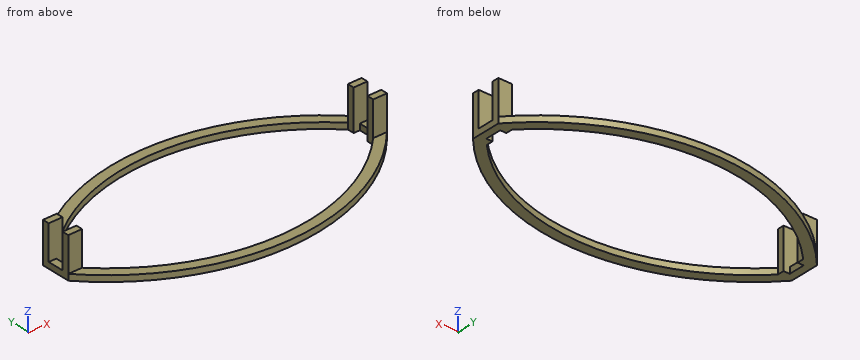
from build123d import *

# Parameters (mm, degrees)
F0_W     = 3.75
F0_H     = 8
F1_DEPTH = 3
F2_DEPTH = 20


with BuildPart() as f1:
    # F0 (on Top) → F1 (new body)
    with BuildSketch(Plane.XY):
        with BuildLine():
            Line((-3.75, 11.307189), (3.051668, 11.307189))
            ThreePointArc((3.051668, 11.307189), (75, 41.856217), (146.948332, 11.307189))
            Line((146.948332, 11.307189), (153.75, 11.307189))
            ThreePointArc((153.75, 11.307189), (75, 46.856217), (-3.75, 11.307189))
        make_face()
        with BuildLine():
            ThreePointArc((146.948332, -3.307189), (75, -33.856217), (3.051668, -3.307189))
            Line((3.051668, -3.307189), (-3.75, -3.307189))
            ThreePointArc((-3.75, -3.307189), (75, -38.856217), (153.75, -3.307189))
            Line((153.75, -3.307189), (146.948332, -3.307189))
        make_face()
        with Locations((151.875, 4)):
            Rectangle(F0_W, F0_H)
        with Locations((-1.875, 4)):
            Rectangle(F0_W, F0_H)
    extrude(amount=F1_DEPTH)

    # F0 (on Top) → F2 (join)
    with BuildSketch(Plane.XY):
        with BuildLine():
            Line((-3.75, 8), (0, 8))
            ThreePointArc((0, 8), (1.507229, 9.670762), (3.051668, 11.307189))
            Line((3.051668, 11.307189), (-3.75, 11.307189))
            Line((-3.75, 11.307189), (-3.75, 8))
        make_face()
        with BuildLine():
            ThreePointArc((3.051668, 11.307189), (1.507229, 9.670762), (0, 8))
            Line((0, 8), (3.051668, 8))
            Line((3.051668, 8), (3.051668, 11.307189))
        make_face()
        with BuildLine():
            ThreePointArc((3.051668, -3.307189), (1.507229, -1.670762), (0, 0))
            Line((0, 0), (-3.75, 0))
            Line((-3.75, 0), (-3.75, -3.307189))
            Line((-3.75, -3.307189), (3.051668, -3.307189))
        make_face()
        with BuildLine():
            Line((3.051668, 0), (0, 0))
            ThreePointArc((0, 0), (1.507229, -1.670762), (3.051668, -3.307189))
            Line((3.051668, -3.307189), (3.051668, 0))
        make_face()
        with BuildLine():
            Line((153.75, 11.307189), (146.948332, 11.307189))
            ThreePointArc((146.948332, 11.307189), (148.492771, 9.670762), (150, 8))
            Line((150, 8), (153.75, 8))
            Line((153.75, 8), (153.75, 11.307189))
        make_face()
        with BuildLine():
            ThreePointArc((150, 8), (148.492771, 9.670762), (146.948332, 11.307189))
            Line((146.948332, 11.307189), (146.948332, 8))
            Line((146.948332, 8), (150, 8))
        make_face()
        with BuildLine():
            ThreePointArc((150, 0), (148.492771, -1.670762), (146.948332, -3.307189))
            Line((146.948332, -3.307189), (153.75, -3.307189))
            Line((153.75, -3.307189), (153.75, 0))
            Line((153.75, 0), (150, 0))
        make_face()
        with BuildLine():
            Line((146.948332, 0), (146.948332, -3.307189))
            ThreePointArc((146.948332, -3.307189), (148.492771, -1.670762), (150, 0))
            Line((150, 0), (146.948332, 0))
        make_face()
    extrude(amount=F2_DEPTH)


solid = f1.part
The listing builds one solid part. Answer for the finished solid, in the listing's coordinates (mm). Give positions to 0.01 mm unless a question says otherwise; leave off trailing zeros. Write each loop counter-clockwise with the first axis right and the second up, starting at its lowest first coordinate (ties: lowest second). Pieces come first, ordered by that corner, then holes.
Item 1: Section A-A, the plane z = 12.25 is taken. Write down the section's boundary in (x, y), plus the area to 3 significant figures.
Item 2: Find the intervals of material crossed by line 1 along X through (y, z) = (8.5, 16.5); line 2 along X through (y, z) = (21, 2); line 3 along Y through (x, z) = (103.5, 1.5), in increasing order.
Item 3: Section B-B, the plane y = 2.5 is taken. Write down the section's boundary in (x, z), plus the area to 3 significant figures.
Item 4: Flat-ended cylindrical pins translate along their axes: P1, Ø8, axis at x = 126, z = 4, coming from the +Y side; P2, Ø4, axis at x = -1.5, y = 4.5, coming from the +Z side; P3, Ø5, axis at y = 31.5, z = 2.5, coming from the +X side. Find the tip coordinate at first contact, or state that the pin passes through.
Item 5: Section C-C, the plane x = 57 is taken. Write down the section's boundary in (y, z), plus the area to 3 significant figures.
Completed:
1. outline: (-3.75, -3.31) - (3.05, -3.31) - (3.05, 0) - (-3.75, 0) - close; (-3.75, 8) - (3.05, 8) - (3.05, 11.31) - (-3.75, 11.31) - close; (146.95, -3.31) - (153.75, -3.31) - (153.75, 0) - (146.95, 0) - close; (146.95, 8) - (153.75, 8) - (153.75, 11.31) - (146.95, 11.31) - close
1. area: 90.0 mm2
2. line 1: x = -3.75 to 3.05, 146.95 to 153.75
2. line 2: x = 6 to 13.88, 136.12 to 144
2. line 3: y = -34.91 to -29.71, 37.71 to 42.91
3. outline: (-3.75, 0) - (0, 0) - (0, 3) - (-3.75, 3) - close; (150, 0) - (153.75, 0) - (153.75, 3) - (150, 3) - close
3. area: 22.5 mm2
4. P1: stops at y = 35.69
4. P2: stops at z = 3
4. P3: stops at x = 133.57
5. outline: (-37.3, 0) - (-32.22, 0) - (-32.22, 3) - (-37.3, 3) - close; (40.22, 0) - (45.3, 0) - (45.3, 3) - (40.22, 3) - close
5. area: 30.5 mm2
